CAD build for the part. Positions are in the model's coordinates, mm. Face numbers are marked on the shaded views. A direction names the side the tool comes from. Give positions to 0.01 mm unless a question says otherwise; leave off trailing zeros. Loops run counter-clockwise (first coordinate to the right, second up) from the corner with the lowest first, then second, coordinate; pieces in that order, holes last.
Item 1: Mould opens along Y. For the marked faces 3, 4, 5 and 6 say: released by +Y, released by -Y, zero draft, split by the parting line, or undercut.
Item 2: Saw through at D-D on x = -93. Give the cut face in (y, z).
Item 3: Saw through at B-B on z = 70.5. Give the cut face in (x, y), plus the area to 3 significant figures.
Item 4: Saw through at C-C on y = -23. Give the cut face in (x, z), plus the area to 3 significant figures.
Item 5: Probe probe 1 along X at (y, z) = (-169.5, 153); probe 2 along Y at (x, z) = (-128.5, 88); probe 3 along Y at (x, z) = (-126.5, 9.5). List the from-to ranges inside material, lowest first.
Item 6: Which spindle directions (+Z, -Z, +X, -X, +Y, -Y) get a long thin tool onto all of the face, cutting with end or side? Do the marked faces 1 and 2. Say none if no direction does.
Item 7: Drop flat-ended pins along their axis: P1, Ø5.5, axis at x = 32, z = 85.5, coming from the +Y side; P2, Ø12, axis at x = -40.5, z = 54, coming from the -Y side; P3, Ø12, axis at x = -75.5, z = 25, coming from the -Y side. Give the stop position or say it passes through.
Item 8: Saw through at A-A on x = -127.5. Give the cut face in (y, z).
from build123d import *

# Parameters (mm, degrees)
INNER_RING_LEFT_SIDE_DEPTH = 170


with BuildPart() as part:
    # Sketch1 → Inner Ring - Left Side (new body)
    with BuildSketch(Plane.XY):
        with BuildLine():
            Line((-100, -111.803398875), (-100, -150))
            Line((-100, -150), (-111.709430585, -146.096856472))
            ThreePointArc((-111.709430585, -146.096856472), (-113.961775712, -146.440459254), (-115, -148.468564717))
            Line((-115, -148.468564717), (-115, -161.531435283))
            ThreePointArc((-115, -161.531435283), (-113.961775712, -163.559540746), (-111.709430585, -163.903143528))
            Line((-111.709430585, -163.903143528), (-100, -160))
            Line((-100, -160), (-100, -225))
            Line((-100, -225), (-175, -225))
            Line((-175, -225), (-175, 0))
            ThreePointArc((-175, 0), (-112.638803261, 133.93095236), (30, 172.409396496))
            Line((30, 172.409396496), (30, 157.409396496))
            Line((30, 157.409396496), (35, 157.409396496))
            Line((35, 157.409396496), (35, 171.464281995))
            ThreePointArc((35, 171.464281995), (37.50401138, 170.934049067), (40, 170.367250374))
            Line((40, 170.367250374), (40, 144.568322948))
            ThreePointArc((40, 144.568322948), (-131.649591483, 71.891481153), (-100, -111.803398875))
        make_face()
    extrude(amount=INNER_RING_LEFT_SIDE_DEPTH)


solid = part.part
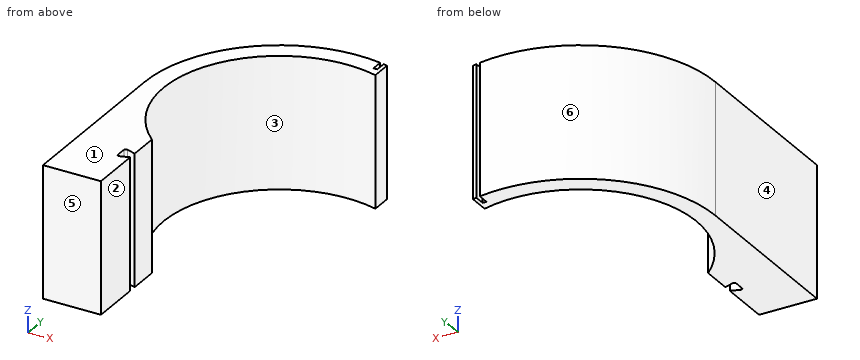
Results below:
1. face 3: undercut
1. face 4: zero draft
1. face 5: released by -Y
1. face 6: released by +Y
2. outline: (117.69, 0) - (148.24, 0) - (148.24, 170) - (117.69, 170) - close
3. outline: (-175, -225) - (-100, -225) - (-100, -160) - (-111.71, -163.9) arc R2.5 cw to (-115, -161.53) - (-115, -148.47) arc R2.5 cw to (-111.71, -146.1) - (-100, -150) - (-100, -111.8) arc R150 cw to (40, 144.57) - (40, 170.37) arc R175 ccw to (35, 171.46) - (35, 157.41) - (30, 157.41) - (30, 172.41) arc R175 ccw to (-175, 0) - close
3. area: 20,100 mm2
4. outline: (-175, 0) - (-148.23, 0) - (-148.23, 170) - (-175, 170) - close
4. area: 4,550 mm2
5. probe 1: x = -175 to -100
5. probe 2: y = -225 to -77.38, 77.38 to 118.8
5. probe 3: y = -225 to -80.61, 80.61 to 120.92
6. face 1: +Z, +X, -X, +Y, -Y
6. face 2: +Z, -Z, +X, -Y
7. P1: stops at y = 172.54
7. P2: stops at y = 142.61
7. P3: stops at y = 125.93
8. outline: (-225, 0) - (-79.02, 0) - (-79.02, 170) - (-225, 170) - close; (79.02, 0) - (119.87, 0) - (119.87, 170) - (79.02, 170) - close
